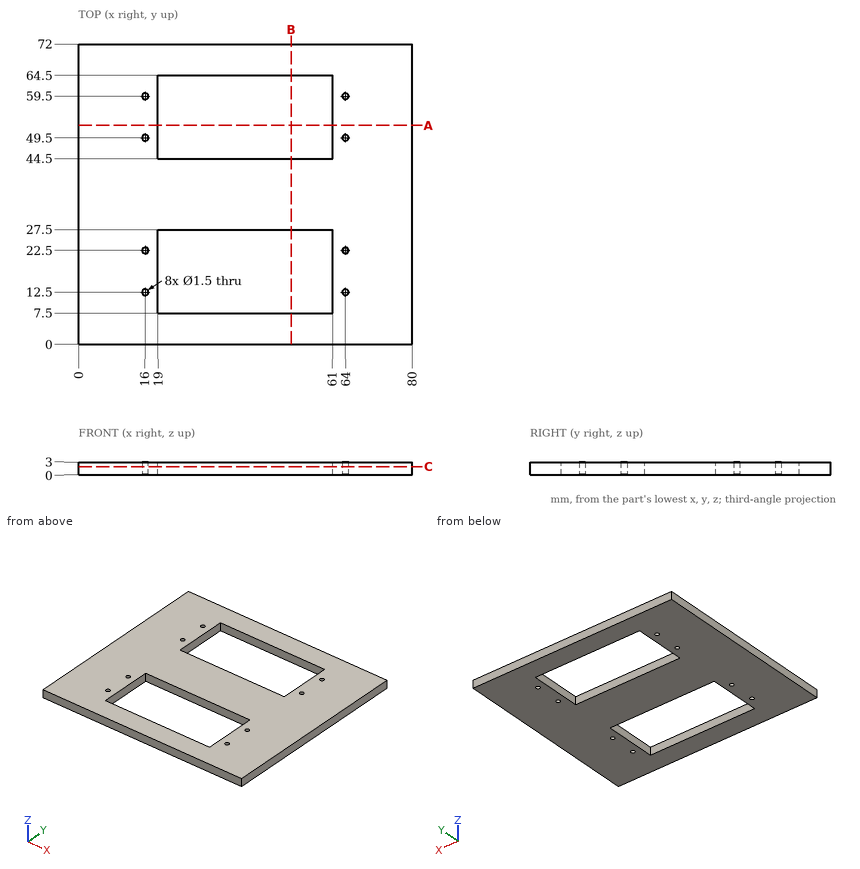
For this review, use the dimensioned drawing (mm, ordinates from the lowest corner) and the shaded views. Round coordinates to 2 decimals unless told otherwise and drop trailing zeros. Order: outer loops, then holes, each group sorted by start corner. A loop starts at its lowest first (then second) coordinate and runs counter-clockwise, first axis right, second up. Notation, with made-up numbers: (-6, 63.5) -> (48, 63.5) arc R21 cw to (48, 67.5) -> close; hole circle Ø11 at (0, -25). An arc over 180 degrees is marked (long way). Write item = value, one per line. Start each with the question number.
Item 1: Consider section C-C on z = 1.95. Count the separate pieces of the cut face and the enclosed holes in it, plus the area to 3 significant figures.
Item 2: For line 1 along X through (y, z) = (22.5, 1.5); line 2 along Y through (x, z) = (33.5, 2.5); line 3 along Y through (x, z) = (16, 0.9), list the stretches that pass through material, from the lowest coordinate up.
Item 3: Consider section B-B on x = 51. Write out the cut boundary in (y, z), plus the area to 3 significant figures.
Item 4: Consider section A-A on y = 52.5. Write out the cut boundary in (x, z), plus the area to 3 significant figures.
Conclusion:
q1.separate_pieces = 1
q1.enclosed_holes = 10
q1.area = 4,070 mm2
q2.line_1 = 0 to 15.25, 16.75 to 19, 61 to 63.25, 64.75 to 80
q2.line_2 = 0 to 7.5, 27.5 to 44.5, 64.5 to 72
q2.line_3 = 0 to 11.75, 13.25 to 21.75, 23.25 to 48.75, 50.25 to 58.75, 60.25 to 72
q3.outline = (0, 0) -> (7.5, 0) -> (7.5, 3) -> (0, 3) -> close; (27.5, 0) -> (44.5, 0) -> (44.5, 3) -> (27.5, 3) -> close; (64.5, 0) -> (72, 0) -> (72, 3) -> (64.5, 3) -> close
q3.area = 96.0 mm2
q4.outline = (0, 0) -> (19, 0) -> (19, 3) -> (0, 3) -> close; (61, 0) -> (80, 0) -> (80, 3) -> (61, 3) -> close
q4.area = 114 mm2
